The model under review builds one solid part; all positions refer to its coordinate system, in mm. A direction names the side the tool comes from. Coordinates: 2 decimals unless noted, no trailing zeros. Loops run counter-clockwise (first coordinate to the right, second up) from the corner with the lowest first, then second, coordinate; pieces in that order, holes last. Notation, with made-up numbers: (-4, 78) - (13, 78) arc R17 ccw to (13, 102) - close; hole circle Ø3 at (-37, 50). An arc over 180 degrees is marked (long way). Use a Markdown table: item, result. Add a question column.
1) For faces 1 (the flat face through (3, 5, 50)), 2 (the flat face through (5, 4, 50)), list the 3-axis set-ups (+Z, -Z, +X, -X, +Y, -Y) from which the entire face can be reached by the end or side of a thin tool; tool diameter is ignored.
2) Add section B-B, the plane z = 53.5. Give the boundary of the cut face in (x, y), and give its area (3 significant figures).
3) Add section A-A, the plane x = 12. Give the boundary of the cut face in (y, z), and give its area (3 significant figures).
4) To check wall thickness, follow L1, parallel to Z at x = 12.25, y = 4.25; L2, parallel to Z at x = 7, y = 4.8; L3, parallel to X at y = 0.95, z = 77.5. State the ranges of each line that lie inside material, in increasing order. Write a range as [from, to].
5) Add section C-C, the plane y = 3.1. Give the boundary of the cut face in (x, z).
6) Clearance check with flat-ended pins moving along their axes: pin 1 (0.8 mm diameter, centred on x = 12.5, y = 4.5, fed in from -Z); pin 2 (1.1 mm diameter, centred on x = 10.5, y = 4.5, fed in from +Z); pin 3 (1.5 mm diameter, centred on y = 3.5, z = 56.5, fed in from +X). State where each tip first meets the part, or that it passes through.
7) Add section D-D, the plane x = 5.5. Give the boundary of the cut face in (y, z).
```python
from build123d import *

# Parameters (mm, degrees)
SALIENTE_EXTRUIR1_DEPTH = 100
CROQUIS2_W              = 7
CROQUIS2_H              = 15
CROQUIS2_W_2            = 12.5
CROQUIS2_H_2            = 40
CORTAR_EXTRUIR1_DEPTH   = 11


with BuildPart() as part:
    # Croquis1 → Saliente-Extruir1 (new body)
    with BuildSketch(Plane.XY):
        Polygon((0, 0), (2, 0), (2, 4), (14.5, 4), (14.5, 5), (2, 5), (0, 5), align=None)
    extrude(amount=SALIENTE_EXTRUIR1_DEPTH)

    # Croquis2 → Cortar-Extruir1 (cut)
    with BuildSketch(Plane(origin=(0, 5, 0), x_dir=(1, 0, 0), z_dir=(0, 1, 0))):
        with Locations((11, -50)):
            Rectangle(CROQUIS2_W, CROQUIS2_H)
        with Locations((8.25, -20)):
            Rectangle(CROQUIS2_W_2, CROQUIS2_H_2)
        with Locations((8.25, -80)):
            Rectangle(CROQUIS2_W_2, CROQUIS2_H_2)
    extrude(amount=-CORTAR_EXTRUIR1_DEPTH, mode=Mode.SUBTRACT)


solid = part.part
```
From the geometry:
| question | item | result |
|---|---|---|
| 1 | face 1 | +Z, -Z, +X, -X, +Y |
| 1 | face 2 | +Z, -Z, +X, -Y |
| 2 | outline | (0, 0) - (2, 0) - (2, 4) - (7.5, 4) - (7.5, 5) - (0, 5) - close |
| 2 | area | 15.5 mm^2 |
| 3 | outline | (4, 40) - (5, 40) - (5, 42.5) - (4, 42.5) - close; (4, 57.5) - (5, 57.5) - (5, 60) - (4, 60) - close |
| 3 | area | 5.00 mm^2 |
| 4 | L1 | z = [40, 42.5], [57.5, 60] |
| 4 | L2 | z = [40, 60] |
| 4 | L3 | x = [0, 2] |
| 5 | outline | (0, 0) - (2, 0) - (2, 100) - (0, 100) - close |
| 6 | pin 1 | stops at z = 40 |
| 6 | pin 2 | stops at z = 60 |
| 6 | pin 3 | stops at x = 7.5 |
| 7 | outline | (4, 40) - (5, 40) - (5, 60) - (4, 60) - close |
